Check sheet for the drawn part. Datum: minimum x, y, z corner. Units: mm. Coordinates: 2 decimals unless noted, no trailing zeros. Write each loop counter-clockwise with the first axis right and the second up, starting at its lowest first coordinate (ties: lowest second). Pieces come first, ordered by that corner, then holes. Notation, with made-up numbers: (21.5, -4) -> (28.5, -4) arc R21 cw to (28.5, 2) -> close; hole circle Ø3 at (88.5, 52). An arc over 180 degrees is marked (long way). Answer in a Markdown table with one row per item.
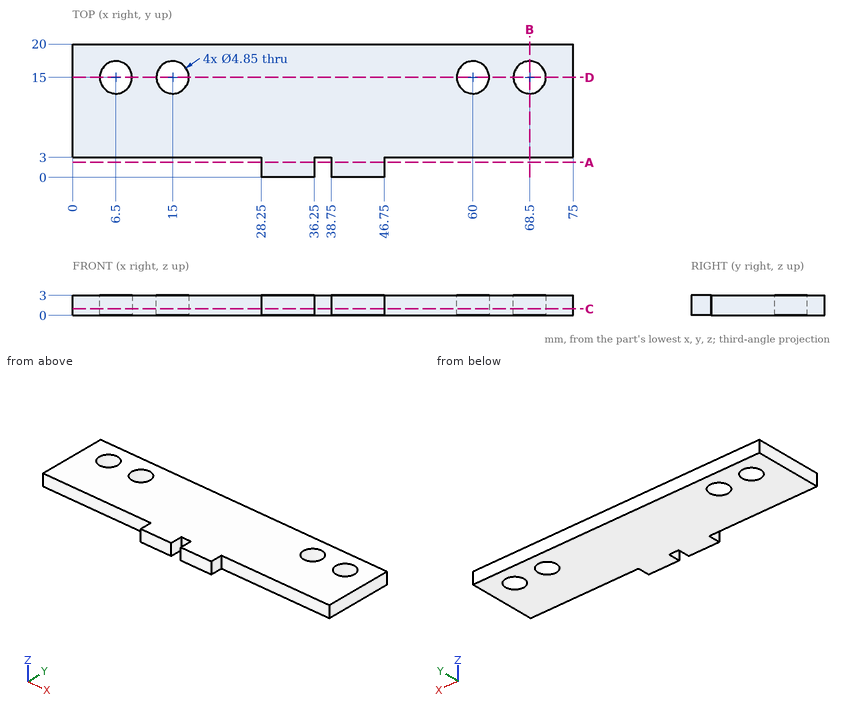
1. Sectioned sample at B-B, the plane x = 68.5. Record the cut outline in (y, z) (3 decimals).
Findings below:
| item | result |
|---|---|
| outline | (3, 0) -> (12.575, 0) -> (12.575, 3) -> (3, 3) -> close; (17.425, 0) -> (20, 0) -> (20, 3) -> (17.425, 3) -> close |
2. Sectioned sample at A-A, the plane y = 2.25. Record the cut outline in (x, z).
Findings below:
| item | result |
|---|---|
| outline | (28.25, 0) -> (36.25, 0) -> (36.25, 3) -> (28.25, 3) -> close; (38.75, 0) -> (46.75, 0) -> (46.75, 3) -> (38.75, 3) -> close |
3. Go/stop test with flat-tipped pins: pin 1 (1.5 mm diameter, centred on y = 1, z = 1.5, fed in from +X); pin 2 (0.9 mm diameter, centred on y = 1, z = 1, fed in from -X); pin 3 (0.8 mm diameter, centred on x = 37, z = 2, fed in from -Y). Record where each tip stops, or that it passes through.
Findings below:
| item | result |
|---|---|
| pin 1 | stops at x = 46.75 |
| pin 2 | stops at x = 28.25 |
| pin 3 | stops at y = 3 |
4. Sectioned sample at C-C, the plane z = 1. Record the cut outline in (x, y) (3 decimals).
Findings below:
| item | result |
|---|---|
| outline | (0, 3) -> (28.25, 3) -> (28.25, 0) -> (36.25, 0) -> (36.25, 3) -> (38.75, 3) -> (38.75, 0) -> (46.75, 0) -> (46.75, 3) -> (75, 3) -> (75, 20) -> (0, 20) -> close; hole circle Ø4.85 at (6.5, 15); hole circle Ø4.85 at (15, 15); hole circle Ø4.85 at (60, 15); hole circle Ø4.85 at (68.5, 15) |
5. Material ranges on probe 1 along Y at (x, z) = (15, 2.1) (3 decimals); probe 2 along Y at (x, z) = (19.5, 2.6); probe 3 along Y at (x, z) = (16.5, 2.55), recorded low to high. Write a range as from..to.
Findings below:
| item | result |
|---|---|
| probe 1 | y = 3..12.575, 17.425..20 |
| probe 2 | y = 3..20 |
| probe 3 | y = 3..13.09, 16.91..20 |
6. Sectioned sample at D-D, the plane y = 15. Record the cut outline in (x, z) (3 decimals), and give its area (3 significant figures).
Findings below:
| item | result |
|---|---|
| outline | (0, 0) -> (4.075, 0) -> (4.075, 3) -> (0, 3) -> close; (8.925, 0) -> (12.575, 0) -> (12.575, 3) -> (8.925, 3) -> close; (17.425, 0) -> (57.575, 0) -> (57.575, 3) -> (17.425, 3) -> close; (62.425, 0) -> (66.075, 0) -> (66.075, 3) -> (62.425, 3) -> close; (70.925, 0) -> (75, 0) -> (75, 3) -> (70.925, 3) -> close |
| area | 167 mm² |
